Design review of the part built by this model. Coordinates are the model's own, in mm. A direction names the side the tool comes from. Give positions to 0.01 mm unless a question says otherwise; leave off trailing zeros. Write each loop counter-clockwise with the first axis right and the second up, starting at its lowest first coordinate (ties: lowest second). Pieces come first, ordered by that corner, then holes. Notation, with made-up numbers: (39.5, 79) -> (86.5, 79) arc R5 cw to (86.5, 85) -> close; hole circle Ø11 at (-27.75, 73). An arc over 180 degrees is marked (long way). Return JSON: item names as keys, results as strings. Group by question number.
from build123d import *

# Parameters (mm, degrees)
SKETCH4_R                    = 5
CUT_EXTRUDE1_DEPTH           = 119.95
SKETCH5_R                    = 7.5
CUT_EXTRUDE2_DEPTH           = 80
M18_TAPPED_HOLE1_D           = 15.5
M18_TAPPED_HOLE1_DEPTH       = 5
M18_TAPPED_HOLE1_CSINK_D     = 18.05
M18_TAPPED_HOLE1_CSINK_ANGLE = 90
M18_TAPPED_HOLE1_TIP         = 4.656669797


with BuildPart() as part:
    # Sketch3 → Revolve2 (revolve)
    with BuildSketch(Plane(origin=(0, 0, 0), x_dir=(0, 0, -1), z_dir=(1, 0, 0))):
        Polygon((0, 12.5), (10, 12.5), (10, 10), (129.95, 10), (129.95, 0), (0, 0), align=None)
    revolve(axis=Axis((0, 0, 0), (0, 0, -1)))

    # Sketch4 → Cut-Extrude1 (cut)
    with BuildSketch(Plane(origin=(0, 0, -129.95), x_dir=(-1, 0, 0), z_dir=(0, 0, -1))):
        Circle(SKETCH4_R)
    extrude(amount=-CUT_EXTRUDE1_DEPTH, mode=Mode.SUBTRACT)

    # Sketch5 → Cut-Extrude2 (cut)
    with BuildSketch(Plane.XY):
        Circle(SKETCH5_R)
    extrude(amount=-CUT_EXTRUDE2_DEPTH, mode=Mode.SUBTRACT)

    # M18 Tapped Hole1
    with Locations(Plane.XY):
        with Locations((0, 0)):
            CounterSinkHole(M18_TAPPED_HOLE1_D / 2, M18_TAPPED_HOLE1_CSINK_D / 2, depth=M18_TAPPED_HOLE1_DEPTH, counter_sink_angle=M18_TAPPED_HOLE1_CSINK_ANGLE)
            with Locations((0, 0, -(M18_TAPPED_HOLE1_DEPTH + M18_TAPPED_HOLE1_TIP / 2))):  # 118° drill point
                Cone(0, M18_TAPPED_HOLE1_D / 2, M18_TAPPED_HOLE1_TIP, mode=Mode.SUBTRACT)


solid = part.part
Q1. Insertion check: pin 1 (4 mm diameter, centred on y = -7.5, z = -103.5, fed in from +X); pin 2 (2 mm diameter, centred on x = 5, z = -27, fed in from -Y); pin 3 (12 mm diameter, centred on x = -5.5, z = -60.5, fed in from -Y); pin 4 (6 mm diameter, centred on x = 0, y = 0, fed in from -Z). Each pin has a flat end and moves straight along its axis. Give the tip position at first contact, or say it passes through.
Q2. Tool access review of faces 1 (the face through (2, -5, -80)), 2 (the face through (7, -6, 0)), 3 (the face through (10.2, -0.1, -10)): name each direction out of +Z, -Z, +X, -X, +Y, -Y from which nothing blocks a thin tool from reaching the whole face with its end or side.
Q3. Mouldability with a two-part tool opening along X and no side actions: class faces 4 (the face through (-9.76, -2.17, -70.81)), 5 (the face through (5, 2, -129.95)), 6 (the face through (1.08, -4.88, -105.32)) as +X half, -X half, draft (parallel to the pull), parting line (faces both ways), or undercut.
Q4. Take a section at C-C, the plane z = -47. Give the boundary of the cut face in (x, y), plus the area to 3 significant figures.
Q5. Take a section at D-D, the plane z = -114. Give the boundary of the cut face in (x, y).
Q6. Take a section at A-A, the plane x = 0. Give the boundary of the cut face in (y, z) (3 decimals), plus the area to 3 significant figures.
Q7. For L1, parallel to Z at x = -7, y = -10; L2, parallel to Y at x = 5.75, z = -72; L3, parallel to X at y = 0, z = -2.35, list the stretches that pass through material, from the lowest coordinate up. Write a range as from..to.
Final values:
{
 "1": {"pin 1": "stops at x = 8.35", "pin 2": "stops at y = -9.17", "pin 3": "stops at y = -10", "pin 4": "passes through"},
 "2": {"face 1": "+Z", "face 2": "+Z, +X, -X, +Y, -Y", "face 3": "-Z"},
 "3": {"face 4": "parting line", "face 5": "draft", "face 6": "undercut"},
 "4": {"outline": "circle Ø20 at (0, 0); hole circle Ø15 at (0, 0)", "area": "137 mm²"},
 "5": {"outline": "circle Ø20 at (0, 0); hole circle Ø10 at (0, 0)"},
 "6": {"outline": "(-12.5, -10) -> (-10, -10) -> (-10, -129.95) -> (-5, -129.95) -> (-5, -80) -> (-7.5, -80) -> (-7.5, -5.15) -> (-7.75, -5) -> (-7.75, -1.275) -> (-9.025, 0) -> (-12.5, 0) -> close; (5, -129.95) -> (10, -129.95) -> (10, -10) -> (12.5, -10) -> (12.5, 0) -> (9.025, 0) -> (7.75, -1.275) -> (7.75, -5) -> (7.5, -5.15) -> (7.5, -80) -> (5, -80) -> close", "area": "945 mm²"},
 "7": {"L1": "z = -10..0", "L2": "y = -8.18..-4.82, 4.82..8.18", "L3": "x = -12.5..-7.75, 7.75..12.5"}
}
